The listing builds one solid part. Answer for the finished solid, in the listing's coordinates (mm). A direction names the side the tool comes from. Coordinates: 2 decimals unless noted, no trailing zeros. Write each loop counter-clockwise with the first axis right and the second up, starting at its lowest first coordinate (ties: lowest second). Pieces come first, ordered by that corner, then holes.
```python
from build123d import *

# Parameters (mm, degrees)
F1_DEPTH = 60
F2_W     = 70
F2_H     = 15
F3_DEPTH = 50
F4_R     = 15
F5_R     = 15
F6_DEPTH = 67.5


with BuildPart() as f1:
    # F0 (on Front) → F1 (new body)
    with BuildSketch(Plane.XZ):
        Polygon((-8.039089, 59.247605), (-48.039089, 59.247605), (-48.039089, -60.752395), (-8.039089, -60.752395), (-8.039089, -20.752395), (11.960911, -20.752395), (11.960911, -60.752395), (51.960911, -60.752395), (51.960911, 59.247605), (11.960911, 59.247605), (11.960911, 19.247605), (-8.039089, 19.247605), align=None)
    extrude(amount=F1_DEPTH)

    # F2 (on face) → F3 (cut)
    with BuildSketch(Plane.XZ.offset(60)):
        with Locations((1.960911, -0.752395)):
            Rectangle(F2_W, F2_H)
    extrude(amount=-F3_DEPTH, mode=Mode.SUBTRACT)

    # F4 (on face) + F5 (on face) → F6 (cut)
    with BuildSketch(Plane(origin=(0, 0, -60.752395), x_dir=(1, 0, 0), z_dir=(0, 0, -1))):
        with Locations((-28.039089, 20)):
            Circle(F4_R)
    with BuildSketch(Plane(origin=(0, 0, -60.752395), x_dir=(1, 0, 0), z_dir=(0, 0, -1))):
        with Locations((31.960911, 20)):
            Circle(F5_R)
    extrude(amount=-F6_DEPTH, mode=Mode.SUBTRACT)


solid = f1.part
```
(1) Each of these flat-tipped pins is pushed along its axis until it touches: pin 1 (7.5 mm diameter, centred on x = 9, z = -2, fed in from -Y); pin 2 (6 mm diameter, centred on x = 5.5, y = -34, fed in from -Z); pin 3 (16 mm diameter, centred on x = 2.5, y = -29, fed in from +Z). Where does it stop, or does it pass through?
(2) For a pull along X with two mould halves and no side action, classify faces 1 (the flat face through (32, -36, -60.752)), 2 (the flat face through (-48.039, -30, 0)), 3 (the flat face through (1, -33, 6.748)) as pulls with the +X half, pulls with the -X half, needs draft (parallel to the pull), parting line crosses it, or undercut.
(3) Which of the six approach directions +Z, -Z, +X, -X, +Y, -Y give full straight-line access (tool end or side, diameter ignored) to faces 4 (the flat face through (-8.039, -30, 39)), 5 (the flat face through (-8.039, -30, -41)), 6 (the flat face through (1, -41, -8.252))?
(4) Find the intervals of material crossed by probe 1 along X at (y, z) = (-20, -10); probe 2 along X at (y, z) = (-20, -39); probe 3 along X at (y, z) = (-9.5, 50.5), in increasing order.
(5) Section B-B, the plane z = 21 is taken. Write down the section's boundary in (x, y), plus the area to 3 significant figures.
(6) Section C-C, the plane x = -6.5 is taken. Write down the section's boundary in (y, z), plus the area to 3 significant figures.
(7) Section A-A, the plane y = -20 is taken. Write down the section's boundary in (x, z), plus the area to 3 significant figures.
(8) Section D-D, the plane x = -20 is taken. Write down the section's boundary in (y, z), plus the area to 3 significant figures.
Solution:
1. pin 1: stops at y = -10
1. pin 2: stops at z = -20.75
1. pin 3: stops at z = 19.25
2. face 1: needs draft
2. face 2: pulls with the -X half
2. face 3: undercut
3. face 4: +Z, +Y, -Y
3. face 5: -Z, +Y, -Y
3. face 6: -Y
4. probe 1: x = -48.04 to -43.04, -13.04 to 16.96, 46.96 to 51.96
4. probe 2: x = -48.04 to -43.04, -13.04 to -8.04, 11.96 to 16.96, 46.96 to 51.96
4. probe 3: x = -48.04 to -8.04, 11.96 to 51.96
5. outline: (-48.04, -60) - (-8.04, -60) - (-8.04, 0) - (-48.04, 0) - close; (11.96, -60) - (51.96, -60) - (51.96, 0) - (11.96, 0) - close
5. area: 4,800 mm2
6. outline: (-60, -20.75) - (0, -20.75) - (0, 19.25) - (-60, 19.25) - (-60, 6.75) - (-10, 6.75) - (-10, -8.25) - (-60, -8.25) - close
6. area: 1,650 mm2
7. outline: (-48.04, -60.75) - (-43.04, -60.75) - (-43.04, 6.75) - (46.96, 6.75) - (46.96, -60.75) - (51.96, -60.75) - (51.96, 59.25) - (11.96, 59.25) - (11.96, 19.25) - (-8.04, 19.25) - (-8.04, 59.25) - (-48.04, 59.25) - close; (-13.04, -60.75) - (-8.04, -60.75) - (-8.04, -20.75) - (11.96, -20.75) - (11.96, -60.75) - (16.96, -60.75) - (16.96, -8.25) - (-13.04, -8.25) - close
7. area: 5,900 mm2
8. outline: (-60, -60.75) - (-32.66, -60.75) - (-32.66, -8.25) - (-60, -8.25) - close; (-60, 6.75) - (-7.34, 6.75) - (-7.34, -60.75) - (0, -60.75) - (0, 59.25) - (-60, 59.25) - close
8. area: 5,080 mm2
